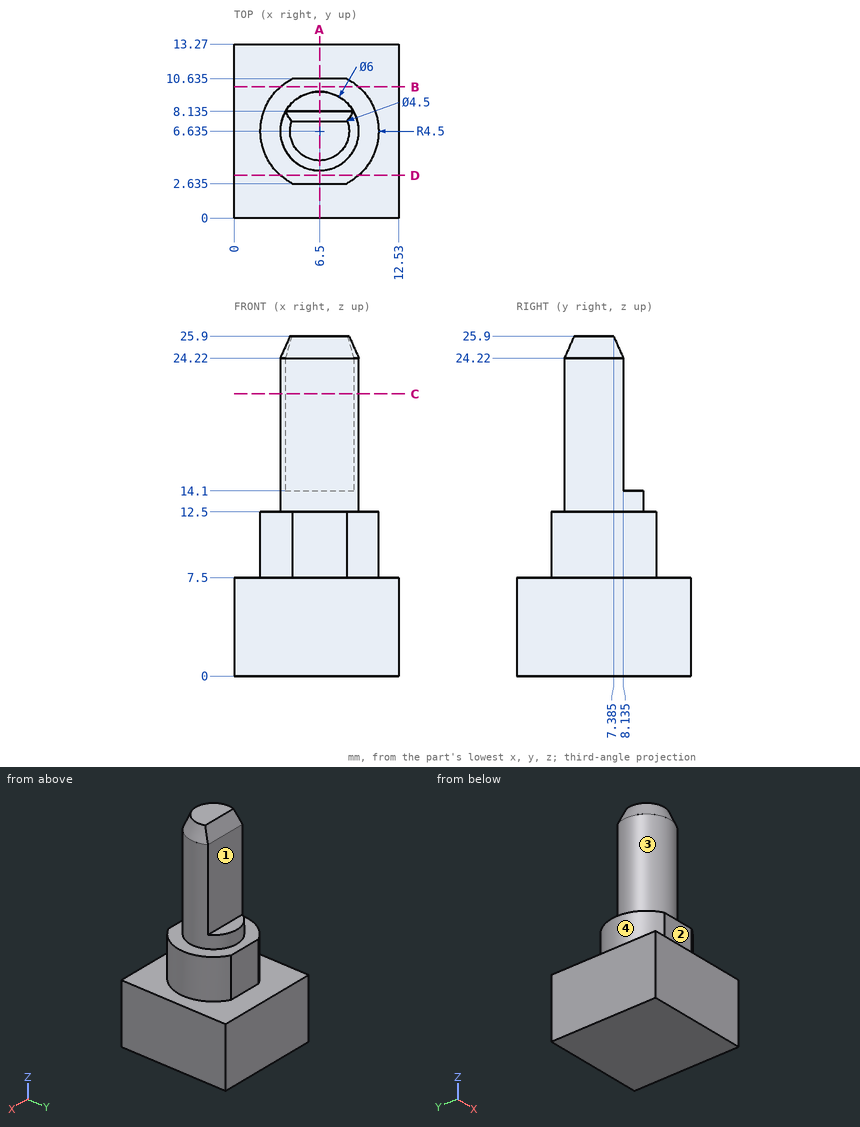
Could you check a few things on this drawing? It's one solid part, dimensions in mm from its lowest x, y, z. A direction names the side the tool comes from. Coordinates: 2 decimals unless noted, no trailing zeros. Order: outer loops, then holes, each group sorted by start corner. A loop starts at its lowest first (then second) coordinate and runs counter-clockwise, first axis right, second up.
1) Imagine slicing it at B-B on y = 10. List the corners of the cut face in (x, z) for me.
2) Imagine slicing it at A-A on x = 6.5. List the corners of the cut face in (y, z) for me (3 decimals).
3) Will these pins go through, and if not, where does the flat tip stop? pin 1 (2 mm diameter, centred on x = 10.5, y = 6.5, fed in from -Z); pin 2 (1.2 mm diameter, centred on x = 6, y = 9, fed in from +Z); pin 3 (1.2 mm diameter, centred on x = 7.5, z = 10, fed in from +Y) (3 decimals); pin 4 (4 mm diameter, centred on x = 7, z = 18, fed in from +Y) (3 decimals).
4) Imagine slicing it at C-C on z = 21.5. List the corners of the cut face in (x, y) for me (3 decimals), and give its area (3 significant figures).
5) Which directions (+Z, -Z, +X, -X, +Y, -Y) give clear straight access to the entire face, cutting with the end or side of a thin tool? Please do the marked faces 1, 2, 3 and 4.
6) I need wall thicknesses on line 1 (Y direction, x = 6.75, z = 11.5) (3 decimals); line 2 (Z direction, x = 4, y = 11.75); line 3 (Z direction, x = 6.5, y = 8.5). Which ranges of each line are inside material? Lowest first, please.
7) Imagine slicing it at D-D on y = 3.25. List the corners of the cut face in (x, z) for me.
Response values:
1. outline: (0, 0) - (12.53, 0) - (12.53, 7.5) - (9.49, 7.5) - (9.49, 12.5) - (3.51, 12.5) - (3.51, 7.5) - (0, 7.5) - close
2. outline: (0, 0) - (13.27, 0) - (13.27, 7.5) - (10.635, 7.5) - (10.635, 12.5) - (9.635, 12.5) - (9.635, 14.1) - (8.135, 14.1) - (8.135, 24.22) - (7.385, 25.9) - (4.385, 25.9) - (3.635, 24.22) - (3.635, 12.5) - (2.635, 12.5) - (2.635, 7.5) - (0, 7.5) - close
3. pin 1: stops at z = 0
3. pin 2: stops at z = 14.1
3. pin 3: stops at y = 10.635
3. pin 4: stops at y = 8.135
4. outline: (3.902, 8.135) arc R3 ccw (long way) to (9.098, 8.135) - close
4. area: 22.7 mm2
5. face 1: +Z, +X, -X, +Y
5. face 2: +Z, +X, -X, -Y
5. face 3: +Z
5. face 4: +Z, -X
6. line 1: y = 2.635 to 10.635
6. line 2: z = 0 to 7.5
6. line 3: z = 0 to 14.1
7. outline: (0, 0) - (12.53, 0) - (12.53, 7.5) - (9.47, 7.5) - (9.47, 12.5) - (3.53, 12.5) - (3.53, 7.5) - (0, 7.5) - close
